```python
from build123d import *

# Parameters (mm, degrees)
SKETCH_1_W          = 2.5
SKETCH_1_H          = 103
SKETCH_1_W_2        = 2
SKETCH_1_H_2        = 95
EXTRUDE_1_DEPTH     = 99.5
CUT_EXTRUDE_2_DEPTH = 4.5
CUT_EXTRUDE_3_DEPTH = 58.5
CUT_EXTRUDE_4_DEPTH = 4.5
SKETCH_6_W          = 1.6
SKETCH_6_H          = 17
CUT_EXTRUDE_5_DEPTH = 10


with BuildPart() as part:
    # 스케치1 → 보스-돌출1 (new body)
    with BuildSketch(Plane(origin=(0, 0, 0), x_dir=(1, 0, 0), z_dir=(0, 1, 0))):
        with Locations((1.25, -51.5)):
            Rectangle(SKETCH_1_W, SKETCH_1_H)
        with Locations((3.5, -51.5)):
            Rectangle(SKETCH_1_W_2, SKETCH_1_H_2)
    extrude(amount=EXTRUDE_1_DEPTH)

    # 스케치2 → 컷-돌출2 (cut)
    with BuildSketch(Plane(origin=(4.5, 0, 0), x_dir=(0, 0, -1), z_dir=(1, 0, 0))):
        with BuildLine():
            Line((-62, 10), (-62, 0))
            Line((-62, 0), (-41, 0))
            Line((-41, 0), (-41, 10))
            ThreePointArc((-41, 10), (-51.5, 20.5), (-62, 10))
        make_face()
    extrude(amount=-CUT_EXTRUDE_2_DEPTH, mode=Mode.SUBTRACT)

    # 스케치3 → 컷-돌출3 (cut)
    with BuildSketch(Plane(origin=(0, 99.5, 0), x_dir=(1, 0, 0), z_dir=(0, 1, 0))):
        Polygon((2.5, -4), (2.5, 0), (0, 0), (0, -103), (2.5, -103), (2.5, -99), (4.5, -99), (4.5, -4), align=None)
    extrude(amount=-CUT_EXTRUDE_3_DEPTH, mode=Mode.SUBTRACT)

    # 스케치4 → 컷-돌출4 (cut)
    with BuildSketch(Plane(origin=(0, 41, 0), x_dir=(1, 0, 0), z_dir=(0, 1, 0))):
        Polygon((4.5, -4), (2.5, -4), (2.5, 0), (0, 0), (0, -103), (2.5, -103), (2.5, -99), (4.5, -99), align=None)
    extrude(amount=-CUT_EXTRUDE_4_DEPTH, mode=Mode.SUBTRACT)

    # 스케치6 → 컷-돌출5 (cut)
    with BuildSketch(Plane.XZ):
        with Locations((0.8, 74)):
            Rectangle(SKETCH_6_W, SKETCH_6_H)
    extrude(amount=-CUT_EXTRUDE_5_DEPTH, mode=Mode.SUBTRACT)


solid = part.part
```
Check sheet for the modelled part. Datum: model origin and axes. Units: mm. A direction names the side the tool comes from. Round coordinates to 2 decimals unless told otherwise and drop trailing zeros. Loops run counter-clockwise (first coordinate to the right, second up) from the corner with the lowest first, then second, coordinate; pieces in that order, holes last. Notation, with made-up numbers: (11, 71) - (30, 71) arc R18 cw to (30, 76) - close; hole circle Ø1 at (37.5, 71). An arc over 180 degrees is marked (long way). Answer as a JSON object with one key per item and string values. Group by question number.
Q1. Sectioned sample at B-B, the plane y = 32.5. Enter the section's corners in (x, z).
Q2. Scan lines: line 1 along Z through (x, y) = (0.5, 6); line 2 along Z through (x, y) = (3.35, 9.5); line 3 along Z through (x, y) = (3.45, 17.5). Record each from-to range of solid material in increasing order. Write a range as [from, to].
Q3. Gauge pin test, flat ends, axial feed: P1, Ø3, axis at y = 25.5, z = 101.5, coming from the +X side; P2, Ø0.5, axis at x = 0.5, z = 71.5, coming from the -Y side; P3, Ø5, axis at y = 4, z = 74.5, coming from the -X side. Record the tip position at first contact, or that the pin passes through.
Q4. Set-up check for faces 1 (the face through (3, 18, 99)), 2 (the face through (2, 5, 41)), 3 (the face through (3, 18, 4)): record each of +Z, -Z, +X, -X, +Y, -Y from which the full face is reachable in a straight line by a thin tool's end or side.
Q5. Sectioned sample at C-C, the plane x = 3.65. Enter the section's corners in (y, z), plus the area to 3 significant figures.
Q6. Sectioned sample at A-A, the plane y = 6. Enter the section's corners in (x, z).
Q7. Sectioned sample at D-D, the plane y = 18. Enter the section's corners in (x, z), plus the area to 3 significant figures.
Solution:
{
 "1": {"outline": "(0, 0) - (2.5, 0) - (2.5, 4) - (4.5, 4) - (4.5, 99) - (2.5, 99) - (2.5, 103) - (0, 103) - close"},
 "2": {"line 1": "z = [0, 41], [62, 65.5], [82.5, 103]", "line 2": "z = [4, 41], [62, 99]", "line 3": "z = [4, 44.15], [58.85, 99]"},
 "3": {"P1": "stops at x = 2.5", "P2": "stops at y = 10", "P3": "stops at x = 1.6"},
 "4": {"face 1": "+Z, +X, +Y, -Y", "face 2": "+X, -X, -Y", "face 3": "-Z, +X, +Y, -Y"},
 "5": {"outline": "(0, 4) - (36.5, 4) - (36.5, 99) - (0, 99) - (0, 62) - (10, 62) arc R10.5 cw to (10, 41) - (0, 41) - close", "area": "3,080 mm²"},
 "6": {"outline": "(0, 0) - (2.5, 0) - (2.5, 4) - (4.5, 4) - (4.5, 41) - (0, 41) - close; (0, 62) - (4.5, 62) - (4.5, 99) - (2.5, 99) - (2.5, 103) - (0, 103) - (0, 82.5) - (1.6, 82.5) - (1.6, 65.5) - (0, 65.5) - close"},
 "7": {"outline": "(0, 0) - (2.5, 0) - (2.5, 4) - (4.5, 4) - (4.5, 44.7) - (0, 44.7) - close; (0, 58.3) - (4.5, 58.3) - (4.5, 99) - (2.5, 99) - (2.5, 103) - (0, 103) - close", "area": "386 mm²"}
}
